Can you work these out from the model? Positions are in its coordinate system, mm. Face numbers are marked on the shaded views. A direction names the side the tool comes from. Give positions to 0.01 mm unless a question says otherwise; leave off trailing zeros. Loops run counter-clockwise (first coordinate to the right, second up) from the corner with the lowest first, then second, coordinate; pieces in that order, holes last. Notation, with made-up numbers: (-35.5, 44) -> (-26.5, 44) arc R15 ccw to (-26.5, 73) -> close; hole circle Ø6 at (43.5, 72). An arc over 180 degrees is marked (long way). Return JSON: item names as keys, results as strings. Group by question number.
Q1. Will these pins go through, and if not, where does the flat tip stop? pin 1 (1 mm diameter, centred on x = -32, y = 54.5, fed in from +Z); pin 2 (5 mm diameter, centred on x = -18, y = 25, fed in from +Z); pin 3 (3 mm diameter, centred on y = 23.5, z = 12, fed in from -X); pin 4 (3 mm diameter, centred on x = -44, y = 66, fed in from +Z).
Q2. Suppose I cut it at B-B, the plane y = 21.5. Please give me the cut outline in (x, z), and give its area (3 significant figures).
Q3. Suppose I cut it at C-C, the plane x = -10.16. Please give me the cut outline in (y, z).
Q4. Suppose I cut it at A-A, the plane z = 45.72. Please give me the cut outline in (x, y).
Q5. I need wall thicknesses on line 1 along X through (y, z) = (55, 45.72); line 2 along Y through (x, z) = (-32.5, 58.5); line 3 along Z through (x, y) = (-10, 54). Which ranges of each line are inside material? Lowest first, please. Write a range as [from, to].
Q6. Suppose I cut it at D-D, the plane z = 69.5. Please give me the cut outline in (x, y), and give its area (3 significant figures).
Q7. Thinking about a two-plate mould opening in Y: for the marked faces 1, 2 and 3, which applies, pulls with the +Y half, pulls with the -Y half, needs draft (parallel to the pull), parting line crosses it, or undercut?
Q8. Which directions (+Z, -Z, +X, -X, +Y, -Y) give clear straight access to the entire face, cutting with the end or side of a thin tool? Please do the marked faces 4 and 5.
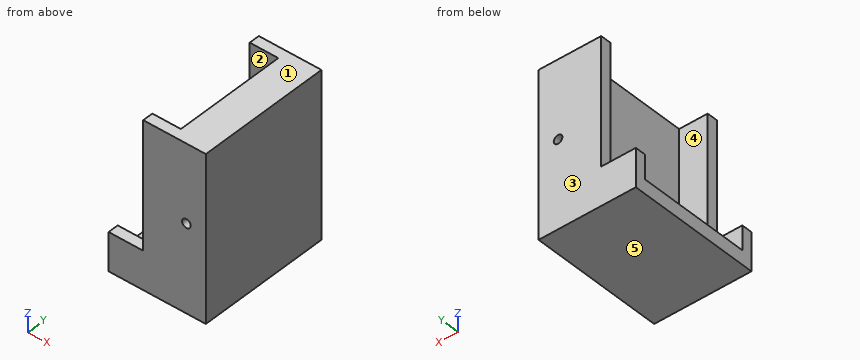
```python
from build123d import *

# Parameters (mm, degrees)
BOSS_EXTRUDE1_DEPTH = 70
SKETCH2_W           = 79
SKETCH2_H           = 59
CUT_EXTRUDE1_DEPTH  = 33.02
SKETCH3_R           = 2.2479
CUT_EXTRUDE2_DEPTH  = 123.22393219


with BuildPart() as part:
    # Sketch1 → Boss-Extrude1 (new body)
    with BuildSketch(Plane(origin=(0, 0, 0), x_dir=(1, 0, 0), z_dir=(0, 1, 0))):
        Polygon((-50.8, -20), (-32.7, -20), (-32.7, -86.36), (0, -86.36), (0, 0), (-50.8, 0), align=None)
    extrude(amount=BOSS_EXTRUDE1_DEPTH)

    # Sketch2 → Cut-Extrude1 (cut)
    with BuildSketch(Plane.ZY.offset(50.8)):
        with Locations((46.86, 35)):
            Rectangle(SKETCH2_W, SKETCH2_H)
    extrude(amount=-CUT_EXTRUDE1_DEPTH, mode=Mode.SUBTRACT)

    # Sketch3 → Cut-Extrude2 (cut, through all)
    with BuildSketch(Plane(origin=(0, 70, 0), x_dir=(1, 0, 0), z_dir=(0, 1, 0))):
        with Locations(Location((-10.16, -45.72, 0), (0, 0, 270))):
            Circle(SKETCH3_R)
    extrude(amount=-CUT_EXTRUDE2_DEPTH, mode=Mode.SUBTRACT)


solid = part.part
```
Ans:
{
 "1": {"pin 1": "stops at z = 7.36", "pin 2": "stops at z = 86.36", "pin 3": "stops at x = -17.78", "pin 4": "stops at z = 20"},
 "2": {"outline": "(-50.8, 0) -> (0, 0) -> (0, 86.36) -> (-17.78, 86.36) -> (-17.78, 7.36) -> (-50.8, 7.36) -> close; hole circle Ø4.5 at (-10.16, 45.72)", "area": "1,760 mm^2"},
 "3": {"outline": "(0, 0) -> (70, 0) -> (70, 43.47) -> (0, 43.47) -> close; (0, 47.97) -> (70, 47.97) -> (70, 86.36) -> (0, 86.36) -> close"},
 "4": {"outline": "(-32.7, 0) -> (-12.41, 0) -> (-12.41, 70) -> (-32.7, 70) -> (-32.7, 64.5) -> (-17.78, 64.5) -> (-17.78, 5.5) -> (-32.7, 5.5) -> close; (-7.91, 0) -> (0, 0) -> (0, 70) -> (-7.91, 70) -> close"},
 "5": {"line 1": "x = [-17.78, -12.41], [-7.91, 0]", "line 2": "y = [0, 5.5], [64.5, 70]", "line 3": "z = [0, 43.48], [47.96, 86.36]"},
 "6": {"outline": "(-32.7, 0) -> (0, 0) -> (0, 70) -> (-32.7, 70) -> (-32.7, 64.5) -> (-17.78, 64.5) -> (-17.78, 5.5) -> (-32.7, 5.5) -> close", "area": "1,410 mm^2"},
 "7": {"face 1": "needs draft", "face 2": "undercut", "face 3": "pulls with the +Y half"},
 "8": {"face 4": "+Z, -X", "face 5": "-Z, +X, -X, +Y, -Y"}
}
